Read the model definition and answer for the solid it produces. Units are mm, in the model's axes. Give positions to 0.01 mm unless a question says otherwise; leave off trailing zeros. Write each loop counter-clockwise with the first axis right and the second up, starting at its lowest first coordinate (ties: lowest second). Pieces come first, ordered by that corner, then holes. Notation, with made-up numbers: (83, 88.25) - (92, 88.25) arc R26 cw to (92, 109.25) - close; hole circle Ø11 at (-34, 56.5). An arc over 180 degrees is marked (long way). Answer as a JSON object with one key per item and string values. Group by question number.
```python
from build123d import *

# Parameters (mm, degrees)
ESBO_O1_W                       = 10
ESBO_O1_H                       = 5.75
RESSALTO_EXTRUS_O1_DEPTH        = 7
ESBO_O2_W                       = 0.6
ESBO_O2_H                       = 0.6
RESSALTO_EXTRUS_O2_DEPTH        = 3.35
CHANFRO1_SIZE                   = 0.1
PADR_O_LINEAR1_COUNT            = 2
PADR_O_LINEAR1_PITCH            = 2.54
CHANFRO1_OF_PADR_O_LINEAR1_SIZE = 0.1
PADR_O_START                    = 0.325
PADR_O_LINEAR2_DEPTH            = 0.4
PADR_O_START_2                  = -2.84
PADR_O_LINEAR2_2_DEPTH          = 0.6
PADR_O_START_3                  = -9.256027766
PADR_O_LINEAR2_3_OUTLINE_W      = 1.336074683
PADR_O_LINEAR2_3_OUTLINE_H      = 1.275
PADR_O_LINEAR2_3_OUTLINE_H_2    = 1.325
PADR_O_LINEAR2_3_DEPTH          = 1.256027766
PADR_O_START_4                  = -10
PADR_O_LINEAR2_4_OUTLINE_W      = 1.663925317
PADR_O_LINEAR2_4_OUTLINE_H      = 1.275
PADR_O_LINEAR2_4_OUTLINE_H_2    = 1.325
PADR_O_LINEAR2_4_DEPTH          = 0.743972234


with BuildPart() as part:
    # Esboço1 → Ressalto-extrusão1 (new body)
    with BuildSketch(Plane.XY):
        Rectangle(ESBO_O1_W, ESBO_O1_H)
    extrude(amount=RESSALTO_EXTRUS_O1_DEPTH)

    # Esboço2 → Ressalto-extrusão2 (add)
    with BuildSketch(Plane.XY.offset(7)):
        with Locations((0, 0.525)):
            Rectangle(ESBO_O2_W, ESBO_O2_H)
    ressalto_extrus_o2 = extrude(amount=RESSALTO_EXTRUS_O2_DEPTH)

    # Chanfro1
    chanfro1_edges = [part.edges().sort_by_distance(p)[0] for p in [
        (0.3, 0.525, 10.35),
        (0, 0.825, 10.35),
        (-0.3, 0.525, 10.35),
        (0, 0.225, 10.35),
    ]]
    chamfer(chanfro1_edges, length=CHANFRO1_SIZE)

    # Padrão linear1: Ressalto-extrusão2 ×2
    with Locations(*[(i * PADR_O_LINEAR1_PITCH, 0, 0) for i in range(1, PADR_O_LINEAR1_COUNT)]):
        add(ressalto_extrus_o2)

    # Chanfro1 of Padrão linear1
    chanfro1_of_padr_o_linear1_edges = [part.edges().sort_by_distance(p)[0] for p in [
        (2.84, 0.525, 10.35),
        (2.54, 0.825, 10.35),
        (2.24, 0.525, 10.35),
        (2.54, 0.225, 10.35),
    ]]
    chamfer(chanfro1_of_padr_o_linear1_edges, length=CHANFRO1_OF_PADR_O_LINEAR1_SIZE)

    # Padrão linear2: read off the stored shape, not the designer's step
    # Padrão linear2 outline → Padrão linear2 (add)
    with BuildSketch(Plane(origin=(0, 0, 0), x_dir=(1, 0, 0), z_dir=(0, 1, 0)).offset(PADR_O_START)):
        Polygon((-2.84, -10.25), (-2.74, -10.35), (-2.34, -10.35), (-2.24, -10.25), (-2.24, -7), (-2.84, -7), align=None)
    extrude(amount=PADR_O_LINEAR2_DEPTH)

    # Padr_o linear2 2 outline → Padr_o linear2 2 (add)
    with BuildSketch(Plane.YZ.offset(PADR_O_START_2)):
        Polygon((0.225, 7), (0.325, 7), (0.325, 10.35), (0.225, 10.25), align=None)
        Polygon((0.825, 7), (0.825, 10.25), (0.725, 10.35), (0.725, 7), align=None)
    extrude(amount=PADR_O_LINEAR2_2_DEPTH)

    # Padr_o linear2 3 outline → Padr_o linear2 3 (cut)
    with BuildSketch(Plane(origin=(0, 0, 0), x_dir=(0.7071067811865471, 0, 0.707106781186548), z_dir=(0.707106781186548, 0, -0.707106781186547)).offset(PADR_O_START_3)):
        with Locations((6.331962659, -1.3625)):
            Rectangle(PADR_O_LINEAR2_3_OUTLINE_W, PADR_O_LINEAR2_3_OUTLINE_H)
        with Locations((6.331962659, 0.3375)):
            Rectangle(PADR_O_LINEAR2_3_OUTLINE_W, PADR_O_LINEAR2_3_OUTLINE_H_2)
    extrude(amount=PADR_O_LINEAR2_3_DEPTH, mode=Mode.SUBTRACT)

    # Padr_o linear2 4 outline → Padr_o linear2 4 (cut)
    with BuildSketch(Plane(origin=(0, 0, 0), x_dir=(0.7071067811865471, 0, 0.707106781186548), z_dir=(0.707106781186548, 0, -0.707106781186547)).offset(PADR_O_START_4)):
        with Locations((4.831962659, -1.3625)):
            Rectangle(PADR_O_LINEAR2_4_OUTLINE_W, PADR_O_LINEAR2_4_OUTLINE_H)
        with Locations((4.831962659, 0.3375)):
            Rectangle(PADR_O_LINEAR2_4_OUTLINE_W, PADR_O_LINEAR2_4_OUTLINE_H_2)
    extrude(amount=PADR_O_LINEAR2_4_DEPTH, mode=Mode.SUBTRACT)


solid = part.part
```
1) Find the intervals of material crossed by line 1 (Z direction, x = 3, y = 1.3), in increasing order. Write a range as [from, to].
2) Find section C-C, the plane x = 3.25. Write down the section's boundary in (y, z) (3 decimals), and give its area (4 significant figures).
3) Find section A-A, the plane z = 9. Write down the section's boundary in (x, y) (3 decimals), and give its area (3 significant figures).
4) Flat-ended cylindrical pins translate along their axes: pin 1 Ø0.5 at (x, z) = (2.5, 8) entering from -Y (3 decimals); pin 2 Ø3 at (x, z) = (1.5, 8) entering from +Y (3 decimals); pin 3 Ø0.7 at (x, z) = (-2.5, 8.5) entering from +Y (3 decimals); pin 4 Ø0.7 at (y, z) = (0.5, 8) entering from -X. Find the tip coordinate at first contact, or state that the pin passes through.
5) Find section B-B, the plane y = -0.65. Write down the section's boundary in (x, z), and give its area (3 significant figures).
Values follow:
{
 "1": {"line 1": "z = [0, 7]"},
 "2": {"outline": "(-2.875, 0) - (2.875, 0) - (2.875, 7) - (-2.875, 7) - close", "area": "40.25 mm2"},
 "3": {"outline": "(-2.84, 0.225) - (-2.24, 0.225) - (-2.24, 0.825) - (-2.84, 0.825) - close; (-0.3, 0.225) - (0.3, 0.225) - (0.3, 0.825) - (-0.3, 0.825) - close; (2.24, 0.225) - (2.84, 0.225) - (2.84, 0.825) - (2.24, 0.825) - close", "area": "1.08 mm2"},
 "4": {"pin 1": "stops at y = 0.225", "pin 2": "stops at y = 2.875", "pin 3": "stops at y = 0.825", "pin 4": "stops at x = -2.84"},
 "5": {"outline": "(-5, 0) - (5, 0) - (5, 7) - (-5, 7) - close", "area": "70.0 mm2"}
}
